Work out the finished part from the listing and answer in its coordinate system (mm). Face numbers are marked on the shaded views. A direction names the side the tool comes from. Round coordinates to 2 decimals unless told otherwise and drop trailing zeros. Write each loop counter-clockwise with the first axis right and the second up, starting at its lowest first coordinate (ties: lowest second). Pieces come first, ordered by that corner, then holes.
from build123d import *

# Parameters (mm, degrees)
F1_DEPTH    = 25.4
F2_SIZE     = 2.54
F3_T1_DEPTH = 120.8411218415
F4_SIZE     = 2.54
F5_W        = 15.5079813242
F5_H        = 16.3934864104
F6_DEPTH    = 25.4
F7_R        = 8.128
F9_D        = 9.525
F9_DEPTH    = 19.05
F9_TIP      = 2.8615986981
F11_D       = 6.477
F11_DEPTH   = 14.2748
F11_TIP     = 1.9458871147


# Not quite as in the source:
# - a fillet or chamfer that OpenCascade refuses, or shapes differently, is made with other operations: its cross-section is extruded or revolved along the edge and cut away or added


with BuildPart() as f1:
    # F0 (on Front) → F1 (new body)
    with BuildSketch(Plane.XZ):
        Polygon((-88.9, 0), (0, 0), (0, 23.7338524312), (-25.4, 23.7338524312), (-25.4, 49.53), (0, 49.53), (0, 73.279), (-88.9, 73.279), align=None)
    extrude(amount=F1_DEPTH)

    # F2
    f2_edges = [f1.edges().sort_by_distance(p)[0] for p in [
        (-44.45, 0, 73.279),
        (0, 0, 61.4045),
        (-88.9, 0, 36.6395),
        (-44.45, 0, 0),
        (0, 0, 11.866926),
    ]]
    chamfer(f2_edges, length=F2_SIZE)

    # F3: chamfer of 19.05 on 2 edges, made by hand

    # F3_s2 → F3_t1 (cut)
    with BuildSketch(Plane.XZ.offset(-46.4505609208)):
        Polygon((-19.05, 73.279), (0, 54.229), (0, 73.279), align=None)
        Polygon((-19.05, 0), (0, 19.05), (0, 0), align=None)
    extrude(amount=F3_T1_DEPTH, mode=Mode.SUBTRACT)

    # F4
    f4_edges = [f1.edges().sort_by_distance(p)[0] for p in [
        (-9.525, 0, 63.754),
        (-9.525, 0, 9.525),
    ]]
    chamfer(f4_edges, length=F4_SIZE)

    # F5 (on face) → F6 (cut)
    with BuildSketch(Plane.XZ.offset(25.4)):
        with Locations((-81.1460093379, 37.0688531548)):
            Rectangle(F5_W, F5_H)
    extrude(amount=-F6_DEPTH, mode=Mode.SUBTRACT)

    # F7
    f7_edges = [f1.edges().sort_by_distance(p)[0] for p in [
        (-73.392019, -12.7, 45.265596),
        (-73.392019, -12.7, 28.87211),
    ]]
    fillet(f7_edges, radius=F7_R)

    # F9
    with Locations(Plane.YZ.offset(-25.4)):
        with Locations((-12.7, 36.6319262156)):
            Hole(F9_D / 2, depth=F9_DEPTH)
            with Locations((0, 0, -(F9_DEPTH + F9_TIP / 2))):  # 118° drill point
                Cone(0, F9_D / 2, F9_TIP, mode=Mode.SUBTRACT)

    # F11
    with Locations(Plane.XZ.offset(25.4)):
        with Locations((-37.4242216349, 36.6319262156)):
            Hole(F11_D / 2, depth=F11_DEPTH)
            with Locations((0, 0, -(F11_DEPTH + F11_TIP / 2))):  # 118° drill point
                Cone(0, F11_D / 2, F11_TIP, mode=Mode.SUBTRACT)


solid = f1.part
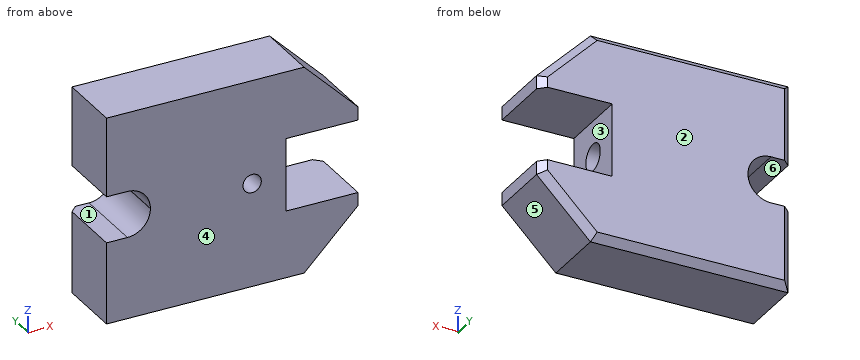
Q1. Find section A-A (y = -4.25). Determine the outline of the cut face in (x, z), plus the area to 3 significant figures.
Q2. Given pin 1 (6 mm diameter, centred on y = -16.5, z = 28, fed in from +X); pin 2 (6 mm diameter, centred on x = -37.42, z = 36.63, fed in from -Y), each flat-ended and moving along its own axis, determine where each tip first touches the part or whether it passes through.
Q3. Find the intervals of material crossed by L1, parallel to Z at x = -24.5, y = -8.75; L2, parallel to Z at x = -36.75, y = -12.7; L3, parallel to X at y = -10.5, z = 47.5, in increasing order.
Q4. Find section C-C (y = -23.5). Determine the outline of the cut face in (x, z).
Q5. The mould has two halves that part along Z. Classify the marked faces 4, 5 and 6: +Z half, -Z half, draft (parallel to the pull), parting line (faces both ways), or undercut.
Q6. Find section B-B (x = -13). Determine the outline of the cut face in (y, z).
Q7. A tool of negligible diameter and unlimited length cuts with its end or side. For the marked faces 1, 2 and 3, from which of +Z, -Z, +X, -X, +Y, -Y can it reach the whole face along a straight path? Write none if from no direction.
Q8. Find section D-D (z = 14.5). Determine the outline of the cut face in (x, y), plus the area to 3 significant figures.
Report:
1. outline: (-88.9, 0) - (-19.05, 0) - (0, 19.05) - (0, 23.73) - (-25.4, 23.73) - (-25.4, 49.53) - (0, 49.53) - (0, 54.23) - (-19.05, 73.28) - (-88.9, 73.28) - (-88.9, 45.27) - (-81.52, 45.27) arc R8.13 cw to (-73.39, 37.14) - (-73.39, 37) arc R8.13 cw to (-81.52, 28.87) - (-88.9, 28.87) - close
1. area: 5,270 mm2
2. pin 1: stops at x = -25.4
2. pin 2: stops at y = -9
3. L1: z = 0 to 23.73, 49.53 to 73.28
3. L2: z = 0 to 31.87, 41.39 to 73.28
3. L3: x = -88.9 to -25.4
4. outline: (-88.9, 0) - (-19.05, 0) - (0, 19.05) - (0, 23.73) - (-25.4, 23.73) - (-25.4, 49.53) - (0, 49.53) - (0, 54.23) - (-19.05, 73.28) - (-88.9, 73.28) - (-88.9, 45.27) - (-81.52, 45.27) arc R8.13 cw to (-73.39, 37.14) - (-73.39, 37) arc R8.13 cw to (-81.52, 28.87) - (-88.9, 28.87) - close; hole circle Ø6.48 at (-37.42, 36.63)
5. face 4: draft
5. face 5: -Z half
5. face 6: undercut
6. outline: (-25.4, 6.05) - (-2.54, 6.05) - (0, 9.64) - (0, 23.73) - (-25.4, 23.73) - close; (-25.4, 49.53) - (0, 49.53) - (0, 63.64) - (-2.54, 67.23) - (-25.4, 67.23) - close
7. face 1: -X, +Y, -Y
7. face 2: +Z, -Z, +X, -X, +Y
7. face 3: +X, +Y, -Y
8. outline: (-88.9, -25.4) - (-4.55, -25.4) - (-4.55, -2.54) - (-8.14, 0) - (-86.36, 0) - (-88.9, -2.54) - close
8. area: 2,130 mm2
